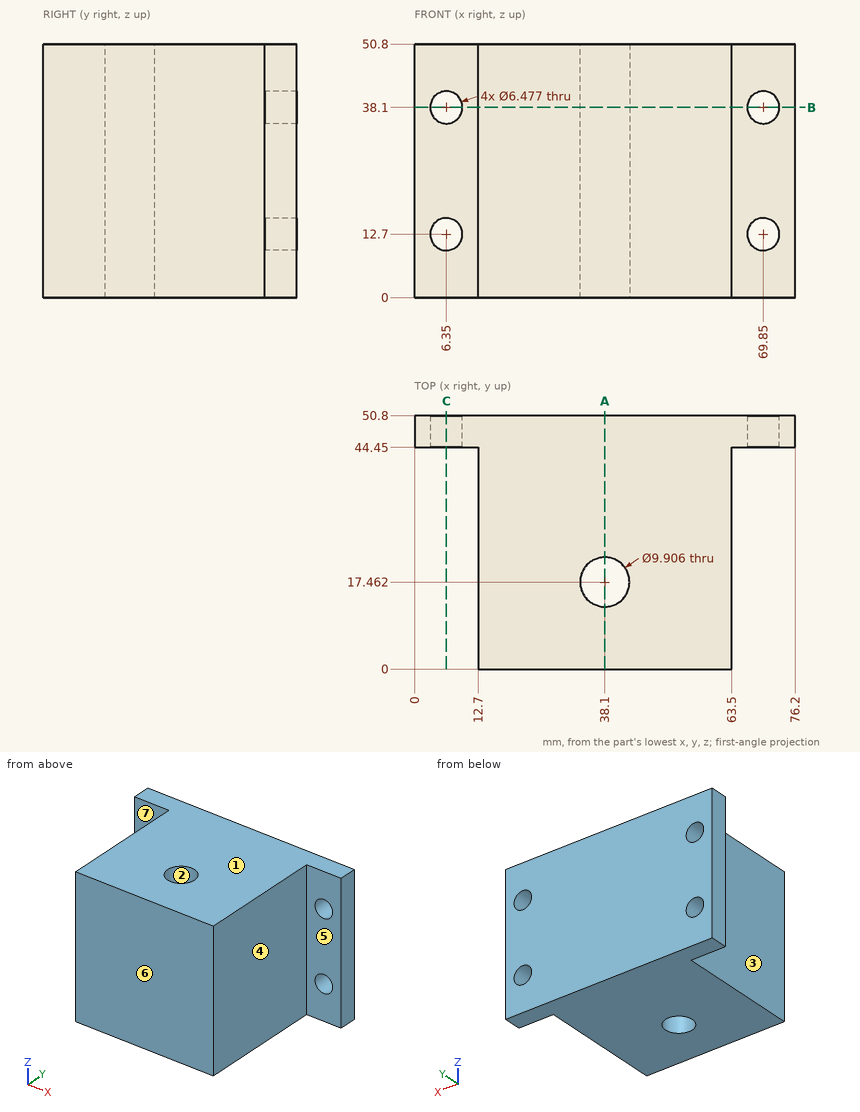
Here's the drawing with two shaded views (mm, measured from the low corner). I have some questions. A direction names the side the tool comes from. Round coordinates to 2 decimals unless told otherwise and drop trailing zeros. Order: outer loops, then holes, each group sorted by start corner. A loop starts at its lowest first (then second) coordinate and runs counter-clockwise, first axis right, second up. Notation, with made-up numbers: M 64,22 L 99,22 A13 ccw 99,35 Z; hole C -20.75,66.25 d11. An arc over 180 degrees is marked long. Use CSV: the item, a comma, the result in double quotes.
1) I'm going to push flat-ended pins straight in: P1, Ø10, axis at x = 4, z = 23.5, coming from the -Y side; P2, Ø6, axis at x = 6.35, z = 12.7, coming from the -Y side; P3, Ø13.5, axis at y = 33, z = 36.5, coming from the -X side; P4, Ø1, axis at y = 27.5, z = 11, coming from the +X side. Where does each tip first touch, or does it pass through?
Taken from the geometry:
P1,"y = 44.45"
P2,"through"
P3,"x = 12.7"
P4,"x = 63.5"
2) I want a section at C-C (x = 6.35). List the corners of the cut face in (y, z) for me, then the cut area to 3 significant figures.
Taken from the geometry:
outline,"M 44.45,0 L 50.8,0 L 50.8,9.46 L 44.45,9.46 Z; M 44.45,15.94 L 50.8,15.94 L 50.8,34.86 L 44.45,34.86 Z; M 44.45,41.34 L 50.8,41.34 L 50.8,50.8 L 44.45,50.8 Z"
area,"240 mm^2"
3) If we mould it in two halves opening along X, with no side actions, what happens to the marked faces 1, 2, 3 and 4? For each: pulls with the +X half, pulls with the -X half, needs draft (parallel to the pull), parting line crosses it, or undercut.
Taken from the geometry:
face 1,"needs draft"
face 2,"undercut"
face 3,"pulls with the -X half"
face 4,"pulls with the +X half"
4) On a 3-axis mill with a long thin cutter (end or side, diameter ignored), from which of +Z, -Z, +X, -X, +Y, -Y can I reach the whole of each face in a straight line? I mean the marked faces 5, 6 and 7. Say none if no direction works.
Taken from the geometry:
face 5,"+Z, -Z, +X, -Y"
face 6,"+Z, -Z, +X, -X, -Y"
face 7,"+Z, -Z, -X, -Y"
5) I want a section at A-A (x = 38.1). List the corners of the cut face in (y, z) for me (1 decimal).
Taken from the geometry:
outline,"M 0,0 L 12.5,0 L 12.5,50.8 L 0,50.8 Z; M 22.4,0 L 50.8,0 L 50.8,50.8 L 22.4,50.8 Z"
6) I want a section at B-B (z = 38.1). Count the separate pieces of the cut face and the enclosed holes in it, then the cut area to 3 significant figures.
Taken from the geometry:
separate pieces,"3"
enclosed holes,"1"
area,"2,580 mm^2"
7) I need wall thicknesses on line 1 along Z through (x, y) = (69.85, 47.5); line 2 along X through (y, z) = (17.5, 23); line 3 along X through (y, z) = (32, 48.5). Which ranges of each line are inside material? Lowest first, please. Write a range as [from, to].
Taken from the geometry:
line 1,"[0, 9.46], [15.94, 34.86], [41.34, 50.8]"
line 2,"[12.7, 33.15], [43.05, 63.5]"
line 3,"[12.7, 63.5]"
